from build123d import *

# Parameters (mm, degrees)
F0_W      = 62
F0_H      = 25
F1_DEPTH  = 1
F3_DEPTH  = 2
F1_FACE_W = 62
F1_FACE_H = 25
F4_DEPTH  = 1


with BuildPart() as f1:
    # F0 (on Top) → F1 (new body)
    with BuildSketch(Plane.XY):
        Rectangle(F0_W, F0_H)
    extrude(amount=F1_DEPTH)

    # F2 (on face) → F3 (join)
    with BuildSketch(Plane.XY.offset(1)):
        with BuildLine():
            Line((-13, 10.5), (-27, 10.5))
            ThreePointArc((-27, 10.5), (-28.414214, 9.914214), (-29, 8.5))
            Line((-29, 8.5), (-29, -10.5))
            Line((-29, -10.5), (-21, -10.5))
            Line((-21, -10.5), (-21, 2.5))
            Line((-21, 2.5), (-19, 2.5))
            Line((-19, 2.5), (-19, -8.5))
            ThreePointArc((-19, -8.5), (-18.414214, -9.914214), (-17, -10.5))
            Line((-17, -10.5), (-3, -10.5))
            ThreePointArc((-3, -10.5), (-1.585786, -9.914214), (-1, -8.5))
            Line((-1, -8.5), (-1, 2.5))
            Line((-1, 2.5), (1, 2.5))
            Line((1, 2.5), (1, -8.5))
            ThreePointArc((1, -8.5), (1.585786, -9.914214), (3, -10.5))
            Line((3, -10.5), (17, -10.5))
            ThreePointArc((17, -10.5), (18.414214, -9.914214), (19, -8.5))
            Line((19, -8.5), (19, 2.5))
            Line((19, 2.5), (21, 2.5))
            Line((21, 2.5), (21, -10.5))
            Line((21, -10.5), (29, -10.5))
            Line((29, -10.5), (29, 8.5))
            ThreePointArc((29, 8.5), (28.414214, 9.914214), (27, 10.5))
            Line((27, 10.5), (13, 10.5))
            ThreePointArc((13, 10.5), (11.585786, 9.914214), (11, 8.5))
            Line((11, 8.5), (11, -2.5))
            Line((11, -2.5), (9, -2.5))
            Line((9, -2.5), (9, 8.5))
            ThreePointArc((9, 8.5), (8.414214, 9.914214), (7, 10.5))
            Line((7, 10.5), (-7, 10.5))
            ThreePointArc((-7, 10.5), (-8.414214, 9.914214), (-9, 8.5))
            Line((-9, 8.5), (-9, -2.5))
            Line((-9, -2.5), (-11, -2.5))
            Line((-11, -2.5), (-11, 8.5))
            ThreePointArc((-11, 8.5), (-11.585786, 9.914214), (-13, 10.5))
        make_face()
    extrude(amount=F3_DEPTH)

    # F1_face (on face) → F4 (cut)
    with BuildSketch(Plane.XY.offset(1)):
        Rectangle(F1_FACE_W, F1_FACE_H)
    extrude(amount=-F4_DEPTH, mode=Mode.SUBTRACT)


solid = f1.part
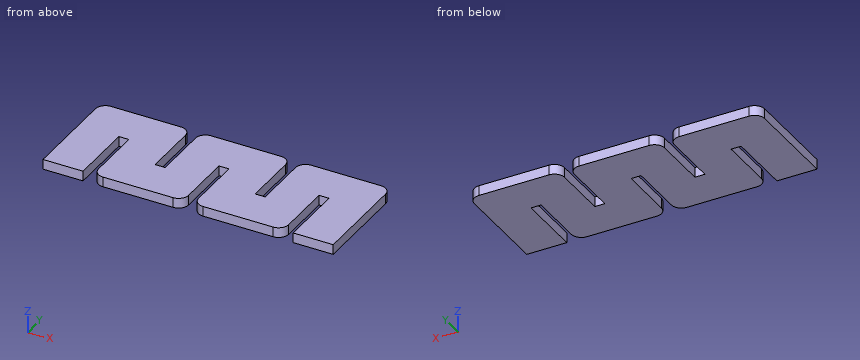
The listing builds one solid part. Answer for the finished solid, in the listing's coordinates (mm). Coordinates: 2 decimals unless noted, no trailing zeros. Order: outer loops, then holes, each group sorted by start corner. A loop starts at its lowest first (then second) coordinate and runs counter-clockwise, first axis right, second up.
Q1. A cutting plane is placed at A-A, the plane y = 3. Write down the section's boundary in (x, z), and give its area (3 significant figures).
Q2. A cutting plane is placed at C-C, the plane x = 20.5. Write down the section's boundary in (y, z), and give its area (3 significant figures).
Q3. A cutting plane is placed at D-D, the plane x = 8.5. Write down the section's boundary in (y, z), and give its area (3 significant figures).
Q4. Consider line 1 (X direction, y = -6, z = 2.6); line 2 (X direction, y = 7.25, z = 2.85); line 3 (X direction, y = -2.25, z = 1.8). Determine where each line is inside the solid, lowest interval first.
Q5. Given P1, Ø0.6, axis at x = -10, z = 2.5, coming from the +Y side, flat-ended and moving along its own axis, determine where the tip first touches the part or whether it passes through.
Answers follow:
1. outline: (-29, 1) - (-11, 1) - (-11, 3) - (-29, 3) - close; (-9, 1) - (9, 1) - (9, 3) - (-9, 3) - close; (11, 1) - (29, 1) - (29, 3) - (11, 3) - close
1. area: 108 mm2
2. outline: (2.5, 1) - (10.5, 1) - (10.5, 3) - (2.5, 3) - close
2. area: 16.0 mm2
3. outline: (-10.5, 1) - (9.82, 1) - (9.82, 3) - (-10.5, 3) - close
3. area: 40.6 mm2
4. line 1: x = -29 to -21, -19 to -1, 1 to 19, 21 to 29
4. line 2: x = -29 to -11, -9 to 9, 11 to 29
4. line 3: x = -29 to -21, -19 to -11, -9 to -1, 1 to 9, 11 to 19, 21 to 29
5. P1: stops at y = -2.5
